```python
from build123d import *

# Parameters (mm, degrees)
SKETCH1_W                = 19
SKETCH1_H                = 110
SKETCH1_W_2              = 3.5
SKETCH1_H_2              = 25
BOSS_EXTRUDE1_DEPTH      = 5
BOSS_EXTRUDE2_DEPTH      = 11.5
BOSS_EXTRUDE2_DEPTH_BACK = 30.5
SKETCH3_R                = 1.5
CUT_EXTRUDE1_DEPTH       = 10
SKETCH4_W                = 4
SKETCH4_H                = 15
BOSS_EXTRUDE3_DEPTH      = 17
BOSS_EXTRUDE4_DEPTH      = 4
FILLET1_R                = 1.5


with BuildPart() as part:
    # Sketch1 → Boss-Extrude1 (new body)
    with BuildSketch(Plane(origin=(0, 0, 0), x_dir=(1, 0, 0), z_dir=(0, 1, 0))):
        with Locations((-9.5, 55)):
            Rectangle(SKETCH1_W, SKETCH1_H)
        with Locations((-9.5, 92.5)):
            Rectangle(SKETCH1_W_2, SKETCH1_H_2, mode=Mode.SUBTRACT)
    extrude(amount=BOSS_EXTRUDE1_DEPTH)

    # Sketch2 → Boss-Extrude2 (add, two sides: drawn at the far end of the back side and taken through both)
    with BuildSketch(Plane(origin=(0, 0, 0), x_dir=(0, 0, -1), z_dir=(1, 0, 0)).offset(-BOSS_EXTRUDE2_DEPTH_BACK)):
        Polygon((10, 15), (10, 35), (0, 35), (0, 15), (0, 5), (0, 0), (10, 0), (10, 5), align=None)
    extrude(amount=BOSS_EXTRUDE2_DEPTH + BOSS_EXTRUDE2_DEPTH_BACK)

    # Sketch3 → Cut-Extrude1 (cut)
    with BuildSketch(Plane(origin=(0, 0, -10), x_dir=(-1, 0, 0), z_dir=(0, 0, -1))):
        with Locations((-8.5, 31)):
            Circle(SKETCH3_R)
        with Locations((-8.5, 23)):
            Circle(SKETCH3_R)
        with Locations((-8.5, 15)):
            Circle(SKETCH3_R)
        with Locations(Location((27.5, 15, 0), (0, 0, 180))):
            Circle(SKETCH3_R)
        with Locations(Location((27.5, 23, 0), (0, 0, 180))):
            Circle(SKETCH3_R)
        with Locations(Location((27.5, 31, 0), (0, 0, 180))):
            Circle(SKETCH3_R)
    extrude(amount=-CUT_EXTRUDE1_DEPTH, mode=Mode.SUBTRACT)

    # Sketch4 → Boss-Extrude3 (add)
    with BuildSketch(Plane(origin=(0, 5, 0), x_dir=(1, 0, 0), z_dir=(0, 1, 0))):
        with Locations((-9.5, 55.5)):
            Rectangle(SKETCH4_W, SKETCH4_H)
    extrude(amount=BOSS_EXTRUDE3_DEPTH)

    # Sketch5 → Boss-Extrude4 (add)
    with BuildSketch(Plane(origin=(-7.5, 0, 0), x_dir=(0, 0, -1), z_dir=(1, 0, 0))):
        with BuildLine():
            Line((63, 22), (68, 22))
            Line((68, 22), (68, 47))
            ThreePointArc((68, 47), (55.5, 42.833333333), (48, 32))
            Line((48, 32), (48, 22))
            Line((48, 22), (63, 22))
        make_face()
    extrude(amount=-BOSS_EXTRUDE4_DEPTH)

    # Fillet1
    fillet1_edges = [part.edges().sort_by_distance(p)[0] for p in [
        (-11.25, 2.5, -105),
        (-11.25, 2.5, -80),
        (-7.75, 2.5, -80),
        (-7.75, 2.5, -105),
        (-19, 2.5, -10),
        (0, 2.5, -10),
        (-30.5, 17.5, -10),
        (-30.5, 17.5, 0),
        (-9.5, 5, -10),
        (11.5, 17.5, 0),
        (11.5, 17.5, -10),
        (-19, 2.5, -110),
        (0, 2.5, -110),
        (-9.5, 32, -48),
        (-9.5, 47, -68),
        (-9.5, 22, -68),
    ]]
    fillet(fillet1_edges, radius=FILLET1_R - 0.0001)  # a hair under: the kernel refuses the full size


solid = part.part
```
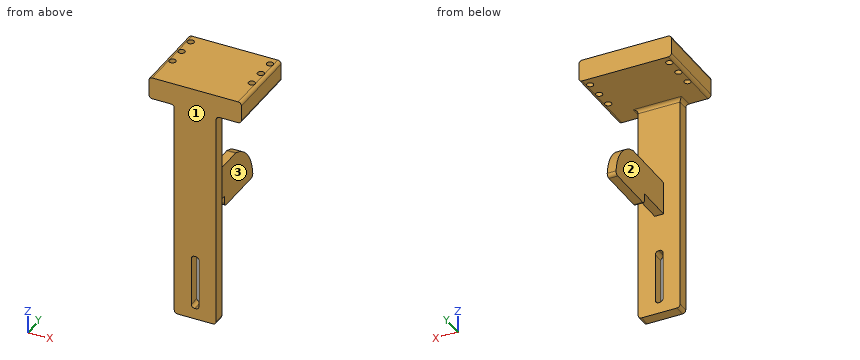
Can you work these out from the model? Positions are in its coordinate system, mm. Face numbers are marked on the shaded views. A direction names the side the tool comes from. Give positions to 0.01 mm unless a question says otherwise; leave off trailing zeros. Loops run counter-clockwise (first coordinate to the right, second up) from the corner with the lowest first, then second, coordinate; pieces in that order, holes last. Notation, with made-up numbers: M 83,45.5 L 112,45.5 A27 ccw 112,83.5 Z; hole C 21,-37 d5. An arc over 180 degrees is marked long. One line per question, with ' | ' between items. Start each with the question number.
Q1. If we section it at B-B (x = 8.5): Please give me the cut outline in (y, z).
Q2. For the marked faces 1, 2 and 3, which set-ups out of +Z, -Z, +X, -X, +Y, -Y let a thin tool reach every point of the face, with its end or its side?
Q3. For pin 1 Ø1.5 at (y, z) = (7, -67.5) entering from -X; pin 2 Ø10 at (x, y) = (-19, 24.5) entering from -Z; pin 3 Ø5.5 at (y, z) = (2.5, -88.5) entering from +X; pin 4 Ø3 at (x, y) = (-9, 38.5) entering from -Z, each with a flat end and sliding along its axis, tell me the tip position at first contact or that it passes through.
Q4. If we section it at A-A (y = 12): Please give me the cut outline in (x, z).
Q5. If we section it at D-D (y = 28): Please give me the cut outline in (x, z).
Q6. If we section it at C-C (z = -98.5): Please give me the cut outline in (x, y).
Q7. If I drill on line 1 (Y direction, x = -27.5, z = -5.5); line 2 (Z direction, x = -22, y = 20.5); line 3 (Y direction, x = -27, z = -4), over which ranges is the centre line in solid material (lowest first)? Write a range as from..to.
Computed:
1) outline: M 0,-10 L 13.5,-10 L 13.5,0 L 0,0 Z; M 16.5,-10 L 21.5,-10 L 21.5,0 L 16.5,0 Z; M 24.5,-10 L 29.5,-10 L 29.5,0 L 24.5,0 Z; M 32.5,-10 L 35,-10 L 35,0 L 32.5,0 Z
2) face 1: +Z, -Z, +X, -X, -Y | face 2: -Z, -X, +Y | face 3: -Z, +X, +Y
3) pin 1: passes through | pin 2: stops at z = -10 | pin 3: stops at x = 0 | pin 4: stops at z = -68
4) outline: M -30.5,-8.5 A1.5 ccw -29,-10 L 10,-10 A1.5 ccw 11.5,-8.5 L 11.5,-1.5 A1.5 ccw 10,0 L -29,0 A1.5 ccw -30.5,-1.5 Z; M -11.5,-63 L -7.5,-63 L -7.5,-48 L -11.5,-48 Z
5) outline: M -30.5,-8.5 A1.5 ccw -29,-10 L 10,-10 A1.5 ccw 11.5,-8.5 L 11.5,-1.5 A1.5 ccw 10,0 L -29,0 A1.5 ccw -30.5,-1.5 Z; M -11.5,-68 L -7.5,-68 L -7.5,-48 L -11.5,-48 Z
6) outline: M -19,0 L -11.25,0 L -11.25,5 L -19,5 Z; M -7.75,0 L 0,0 L 0,5 L -7.75,5 Z
7) line 1: y = 0..13.5, 16.5..21.5, 24.5..29.5, 32.5..35 | line 2: z = -10..0 | line 3: y = 0..13.59, 16.41..21.59, 24.41..29.59, 32.41..35
